Check sheet for the modelled part. Datum: model origin and axes. Units: mm. A direction names the side the tool comes from. Round coordinates to 2 decimals unless told otherwise and drop trailing zeros. Order: outer loops, then holes, each group sorted by start corner. A loop starts at its lowest first (then second) coordinate and runs counter-clockwise, first axis right, second up.
from build123d import *

# Parameters (mm, degrees)
CYLINDER003_R     = 2.125
CYLINDER003_DEPTH = 5
CYLINDER005_R     = 2.125
CYLINDER005_DEPTH = 5
CYLINDER004_R     = 2.125
CYLINDER004_DEPTH = 5
CYLINDER002_R     = 2.125
CYLINDER002_DEPTH = 5
CYLINDER001_R     = 2.125
CYLINDER001_DEPTH = 5
CYLINDER006_R     = 2.125
CYLINDER006_DEPTH = 5
CYLINDER007_R     = 2.125
CYLINDER007_DEPTH = 5
CYLINDER_R        = 2.12
CYLINDER_DEPTH    = 5
BOX_W             = 29
BOX_H             = 15
BOX_DEPTH         = 10


with BuildPart() as cylinder003:
    # Cylinder003 → Cylinder003 (new body)
    with BuildSketch(Plane(origin=(4, 11, 5), x_dir=(1, 0, 0), z_dir=(0, 0, 1))):
        Circle(CYLINDER003_R)
    extrude(amount=CYLINDER003_DEPTH)


with BuildPart() as cylinder005:
    # Cylinder005 → Cylinder005 (new body)
    with BuildSketch(Plane(origin=(25, 4, 5), x_dir=(1, 0, 0), z_dir=(0, 0, 1))):
        Circle(CYLINDER005_R)
    extrude(amount=CYLINDER005_DEPTH)


with BuildPart() as cylinder004:
    # Cylinder004 → Cylinder004 (new body)
    with BuildSketch(Plane(origin=(18, 11, 5), x_dir=(1, 0, 0), z_dir=(0, 0, 1))):
        Circle(CYLINDER004_R)
    extrude(amount=CYLINDER004_DEPTH)


with BuildPart() as cylinder002:
    # Cylinder002 → Cylinder002 (new body)
    with BuildSketch(Plane(origin=(11, 11, 5), x_dir=(1, 0, 0), z_dir=(0, 0, 1))):
        Circle(CYLINDER002_R)
    extrude(amount=CYLINDER002_DEPTH)


with BuildPart() as cylinder001:
    # Cylinder001 → Cylinder001 (new body)
    with BuildSketch(Plane(origin=(11, 4, 5), x_dir=(1, 0, 0), z_dir=(0, 0, 1))):
        Circle(CYLINDER001_R)
    extrude(amount=CYLINDER001_DEPTH)


with BuildPart() as cylinder006:
    # Cylinder006 → Cylinder006 (new body)
    with BuildSketch(Plane(origin=(18, 4, 5), x_dir=(1, 0, 0), z_dir=(0, 0, 1))):
        Circle(CYLINDER006_R)
    extrude(amount=CYLINDER006_DEPTH)


with BuildPart() as cylinder007:
    # Cylinder007 → Cylinder007 (new body)
    with BuildSketch(Plane(origin=(25, 11, 5), x_dir=(1, 0, 0), z_dir=(0, 0, 1))):
        Circle(CYLINDER007_R)
    extrude(amount=CYLINDER007_DEPTH)


with BuildPart() as fusion:
    # Cylinder → Cylinder (new body)
    with BuildSketch(Plane(origin=(4, 4, 5), x_dir=(1, 0, 0), z_dir=(0, 0, 1))):
        Circle(CYLINDER_R)
    extrude(amount=CYLINDER_DEPTH)

    # Fusion: union Cylinder003, Cylinder005, Cylinder004, Cylinder002, Cylinder001, Cylinder006, Cylinder007
    add(cylinder003.part)
    add(cylinder005.part)
    add(cylinder004.part)
    add(cylinder002.part)
    add(cylinder001.part)
    add(cylinder006.part)
    add(cylinder007.part)


with BuildPart() as cut:
    # Box → Box (new body)
    with BuildSketch(Plane.XY):
        with Locations((14.5, 7.5)):
            Rectangle(BOX_W, BOX_H)
    extrude(amount=BOX_DEPTH)

    # Cut: cut Fusion
    add(fusion.part, mode=Mode.SUBTRACT)


solid = cut.part
1) Sectioned sample at B-B on x = 25. Record the cut outline in (y, z) (3 decimals).
2) Scan lines: line 1 (Y direction, x = 11, z = 7.95) (3 decimals); line 2 (X direction, y = 5.75, z = 9.5); line 3 (Y direction, x = 5, z = 8.5) (3 decimals). Record each from-to range of solid material in increasing order.
3) Set-up check for faces 5 (the face through (9.31, 9.71, 7.46)), 6 (the face through (0, 7, 5)): record each of +Z, -Z, +X, -X, +Y, -Y from which the full face is reachable in a straight line by a thin tool's end or side.
4) Sectioned sample at C-C on y = 4. Record the cut outline in (x, z) (3 decimals).
5) Sectioned sample at D-D on x = 4. Record the cut outline in (y, z) (3 decimals), and give its area (3 significant figures).
6) Draft check along Y on faces 1 (the face through (25, 4, 5)), 2 (the face through (14, 8, 10)), 3 (the face through (15.877, 11.093, 7.465)), 4 (the face through (14, 15, 5)). Enter one of: pulls with the +Y half, pulls with the -Y half, needs draft (parallel to the pull), parting line crosses it, or undercut.
7) Sectioned sample at A-A on z = 8.75. Count the separate pieces of the cut face and the enclosed holes in it, and give its area (3 significant figures).
8) Gauge pin test, flat end, axial feed: pin 1 (1.3 mm diameter, centred on x = 4.5, y = 3, fed in from +Z). Record the tip position at first contact, or that the pin passes through.
Values found:
1. outline: (0, 0) - (15, 0) - (15, 10) - (13.125, 10) - (13.125, 5) - (8.875, 5) - (8.875, 10) - (6.125, 10) - (6.125, 5) - (1.875, 5) - (1.875, 10) - (0, 10) - close
2. line 1: y = 0 to 1.875, 6.125 to 8.875, 13.125 to 15
2. line 2: x = 0 to 2.8, 5.2 to 9.79, 12.21 to 16.79, 19.21 to 23.79, 26.21 to 29
2. line 3: y = 0 to 2.131, 5.869 to 9.125, 12.875 to 15
3. face 5: +Z
3. face 6: +Z, -Z, -X, +Y, -Y
4. outline: (0, 0) - (29, 0) - (29, 10) - (27.125, 10) - (27.125, 5) - (22.875, 5) - (22.875, 10) - (20.125, 10) - (20.125, 5) - (15.875, 5) - (15.875, 10) - (13.125, 10) - (13.125, 5) - (8.875, 5) - (8.875, 10) - (6.12, 10) - (6.12, 5) - (1.88, 5) - (1.88, 10) - (0, 10) - close
5. outline: (0, 0) - (15, 0) - (15, 10) - (13.125, 10) - (13.125, 5) - (8.875, 5) - (8.875, 10) - (6.12, 10) - (6.12, 5) - (1.88, 5) - (1.88, 10) - (0, 10) - close
5. area: 108 mm2
6. face 1: undercut
6. face 2: needs draft
6. face 3: undercut
6. face 4: pulls with the +Y half
7. separate pieces: 1
7. enclosed holes: 8
7. area: 322 mm2
8. pin 1: stops at z = 5
